Geometry: final body of the model. Coordinates: model frame, mm. Coordinates: 2 decimals unless noted, no trailing zeros. Order: outer loops, then holes, each group sorted by start corner. A loop starts at its lowest first (then second) coordinate and runs counter-clockwise, first axis right, second up. Notation, with made-up numbers: (41, -39.5) -> (50, -39.5) arc R11 cw to (50, -23.5) -> close; hole circle Ø11 at (-22, -8.75). An arc over 180 degrees is marked (long way). Answer in a Markdown table with one row per item. Add a question column.
1) Section query C-C on x = 30. Return the cut outline in (y, z).
2) Section query D-D on y = 174.5. Return the cut outline in (x, z), then the cut area to 3 significant figures.
3) Ray query, line 1 (Y direction, x = 7, z = 4.55); line 2 (X direction, y = 161.5, z = 2.9); line 3 (X direction, y = 85, z = 3.6). Return the intervals inside material, ascending. Write a range as from..to.
4) Section query B-B on x = -4. Return the cut outline in (y, z).
5) Section query A-A on y = 145. Return the cut outline in (x, z).
```python
from build123d import *

# Parameters (mm, degrees)
SKETCH1_W           = 70
SKETCH1_H           = 130
SKETCH1_W_2         = 5
SKETCH1_H_2         = 25
SKETCH1_W_3         = 5.5
SKETCH1_H_3         = 34.894660298
BOSS_EXTRUDE1_DEPTH = 5
CUT_EXTRUDE1_REACH  = 205.568
SKETCH2_W           = 4.8
SKETCH2_H           = 8
SKETCH2_H_2         = 30
SKETCH2_W_2         = 8
SKETCH2_H_3         = 2
SKETCH2_W_3         = 20
SKETCH2_W_4         = 12
SKETCH2_H_4         = 22
CUT_EXTRUDE2_REACH  = 205.568
SKETCH4_R           = 0.4


with BuildPart() as part:
    # Sketch1 → Boss-Extrude1 (new body)
    with BuildSketch(Plane.XY):
        with Locations((0, 135.474649456)):
            Rectangle(SKETCH1_W, SKETCH1_H)
        with Locations((0, 184.474649456)):
            Rectangle(SKETCH1_W_2, SKETCH1_H_2, mode=Mode.SUBTRACT)
        with Locations((0, 117.579989158)):
            Rectangle(SKETCH1_W_2, SKETCH1_H_2, mode=Mode.SUBTRACT)
        with Locations((0, 151.027319307)):
            Rectangle(SKETCH1_W_3, SKETCH1_H_3, mode=Mode.SUBTRACT)
    extrude(amount=BOSS_EXTRUDE1_DEPTH)

    # Sketch2 → Cut-Extrude1 (cut, up to next)
    with BuildSketch(Plane.XY.offset(5), mode=Mode.PRIVATE) as cut_extrude1_sk1:
        with Locations((-31, 189.474649456)):
            Rectangle(SKETCH2_W, SKETCH2_H)
    cut_extrude1_tool1 = extrude(cut_extrude1_sk1.sketch, amount=-CUT_EXTRUDE1_REACH, mode=Mode.PRIVATE) & part.part
    # Sketch2 → Cut-Extrude1 (cut, up to next)
    with BuildSketch(Plane.XY.offset(5), mode=Mode.PRIVATE) as cut_extrude1_sk2:
        with Locations((-31, 150.474649456)):
            Rectangle(SKETCH2_W, SKETCH2_H_2)
    cut_extrude1_tool2 = extrude(cut_extrude1_sk2.sketch, amount=-CUT_EXTRUDE1_REACH, mode=Mode.PRIVATE) & part.part
    # Sketch2 → Cut-Extrude1 (cut, up to next)
    with BuildSketch(Plane.XY.offset(5), mode=Mode.PRIVATE) as cut_extrude1_sk3:
        with Locations((-31, 81.474649456)):
            Rectangle(SKETCH2_W, SKETCH2_H)
    cut_extrude1_tool3 = extrude(cut_extrude1_sk3.sketch, amount=-CUT_EXTRUDE1_REACH, mode=Mode.PRIVATE) & part.part
    # Sketch2 → Cut-Extrude1 (cut, up to next)
    with BuildSketch(Plane.XY.offset(5), mode=Mode.PRIVATE) as cut_extrude1_sk4:
        with Locations((31, 81.474649456)):
            Rectangle(SKETCH2_W, SKETCH2_H)
    cut_extrude1_tool4 = extrude(cut_extrude1_sk4.sketch, amount=-CUT_EXTRUDE1_REACH, mode=Mode.PRIVATE) & part.part
    # Sketch2 → Cut-Extrude1 (cut, up to next)
    with BuildSketch(Plane.XY.offset(5), mode=Mode.PRIVATE) as cut_extrude1_sk5:
        with Locations((31, 150.474649456)):
            Rectangle(SKETCH2_W, SKETCH2_H_2)
    cut_extrude1_tool5 = extrude(cut_extrude1_sk5.sketch, amount=-CUT_EXTRUDE1_REACH, mode=Mode.PRIVATE) & part.part
    # Sketch2 → Cut-Extrude1 (cut, up to next)
    with BuildSketch(Plane.XY.offset(5), mode=Mode.PRIVATE) as cut_extrude1_sk6:
        with Locations((31, 189.474649456)):
            Rectangle(SKETCH2_W, SKETCH2_H)
    cut_extrude1_tool6 = extrude(cut_extrude1_sk6.sketch, amount=-CUT_EXTRUDE1_REACH, mode=Mode.PRIVATE) & part.part
    # Sketch2 → Cut-Extrude1 (cut, up to next)
    with BuildSketch(Plane.XY.offset(5), mode=Mode.PRIVATE) as cut_extrude1_sk7:
        Polygon((10, 196.974649456), (10, 198.974649456), (-10, 198.974649456), (-10, 196.974649456), (-2.5, 196.974649456), (2.5, 196.974649456), align=None)
    cut_extrude1_tool7 = extrude(cut_extrude1_sk7.sketch, amount=-CUT_EXTRUDE1_REACH, mode=Mode.PRIVATE) & part.part
    # Sketch2 → Cut-Extrude1 (cut, up to next)
    with BuildSketch(Plane.XY.offset(5), mode=Mode.PRIVATE) as cut_extrude1_sk8:
        with Locations((29.4, 197.974649456)):
            Rectangle(SKETCH2_W_2, SKETCH2_H_3)
    cut_extrude1_tool8 = extrude(cut_extrude1_sk8.sketch, amount=-CUT_EXTRUDE1_REACH, mode=Mode.PRIVATE) & part.part
    # Sketch2 → Cut-Extrude1 (cut, up to next)
    with BuildSketch(Plane.XY.offset(5), mode=Mode.PRIVATE) as cut_extrude1_sk9:
        with Locations((-29.4, 197.974649456)):
            Rectangle(SKETCH2_W_2, SKETCH2_H_3)
    cut_extrude1_tool9 = extrude(cut_extrude1_sk9.sketch, amount=-CUT_EXTRUDE1_REACH, mode=Mode.PRIVATE) & part.part
    # Sketch2 → Cut-Extrude1 (cut, up to next)
    with BuildSketch(Plane.XY.offset(5), mode=Mode.PRIVATE) as cut_extrude1_sk10:
        with Locations((-29.4, 72.974649456)):
            Rectangle(SKETCH2_W_2, SKETCH2_H_3)
    cut_extrude1_tool10 = extrude(cut_extrude1_sk10.sketch, amount=-CUT_EXTRUDE1_REACH, mode=Mode.PRIVATE) & part.part
    # Sketch2 → Cut-Extrude1 (cut, up to next)
    with BuildSketch(Plane.XY.offset(5), mode=Mode.PRIVATE) as cut_extrude1_sk11:
        with Locations((0, 72.974649456)):
            Rectangle(SKETCH2_W_3, SKETCH2_H_3)
    cut_extrude1_tool11 = extrude(cut_extrude1_sk11.sketch, amount=-CUT_EXTRUDE1_REACH, mode=Mode.PRIVATE) & part.part
    # Sketch2 → Cut-Extrude1 (cut, up to next)
    with BuildSketch(Plane.XY.offset(5), mode=Mode.PRIVATE) as cut_extrude1_sk12:
        with Locations((29.4, 72.974649456)):
            Rectangle(SKETCH2_W_2, SKETCH2_H_3)
    cut_extrude1_tool12 = extrude(cut_extrude1_sk12.sketch, amount=-CUT_EXTRUDE1_REACH, mode=Mode.PRIVATE) & part.part
    # Sketch2 → Cut-Extrude1 (cut, up to next)
    with BuildSketch(Plane.XY.offset(5), mode=Mode.PRIVATE) as cut_extrude1_sk13:
        with Locations((10, 95.474649456)):
            Rectangle(SKETCH2_W_4, SKETCH2_H_4)
    cut_extrude1_tool13 = extrude(cut_extrude1_sk13.sketch, amount=-CUT_EXTRUDE1_REACH, mode=Mode.PRIVATE) & part.part
    add(cut_extrude1_tool1.solids().sort_by_distance((-31, 189.474649, 5))[0], mode=Mode.SUBTRACT)
    add(cut_extrude1_tool2.solids().sort_by_distance((-31, 150.474649, 5))[0], mode=Mode.SUBTRACT)
    add(cut_extrude1_tool3.solids().sort_by_distance((-31, 81.474649, 5))[0], mode=Mode.SUBTRACT)
    add(cut_extrude1_tool4.solids().sort_by_distance((31, 81.474649, 5))[0], mode=Mode.SUBTRACT)
    add(cut_extrude1_tool5.solids().sort_by_distance((31, 150.474649, 5))[0], mode=Mode.SUBTRACT)
    add(cut_extrude1_tool6.solids().sort_by_distance((31, 189.474649, 5))[0], mode=Mode.SUBTRACT)
    add(cut_extrude1_tool7.solids().sort_by_distance((0, 197.974649, 5))[0], mode=Mode.SUBTRACT)
    add(cut_extrude1_tool8.solids().sort_by_distance((29.4, 197.974649, 5))[0], mode=Mode.SUBTRACT)
    add(cut_extrude1_tool9.solids().sort_by_distance((-29.4, 197.974649, 5))[0], mode=Mode.SUBTRACT)
    add(cut_extrude1_tool10.solids().sort_by_distance((-29.4, 72.974649, 5))[0], mode=Mode.SUBTRACT)
    add(cut_extrude1_tool11.solids().sort_by_distance((0, 72.974649, 5))[0], mode=Mode.SUBTRACT)
    add(cut_extrude1_tool12.solids().sort_by_distance((29.4, 72.974649, 5))[0], mode=Mode.SUBTRACT)
    add(cut_extrude1_tool13.solids().sort_by_distance((10, 95.474649, 5))[0], mode=Mode.SUBTRACT)

    # Sketch4 → Cut-Extrude2 (cut, up to next)
    with BuildSketch(Plane.XY.offset(5), mode=Mode.PRIVATE) as cut_extrude2_sk1:
        with Locations((10, 81.974649456)):
            Circle(SKETCH4_R)
    cut_extrude2_tool1 = extrude(cut_extrude2_sk1.sketch, amount=-CUT_EXTRUDE2_REACH, mode=Mode.PRIVATE) & part.part
    # Sketch4 → Cut-Extrude2 (cut, up to next)
    with BuildSketch(Plane.XY.offset(5), mode=Mode.PRIVATE) as cut_extrude2_sk2:
        with Locations((10, 108.974649456)):
            Circle(SKETCH4_R)
    cut_extrude2_tool2 = extrude(cut_extrude2_sk2.sketch, amount=-CUT_EXTRUDE2_REACH, mode=Mode.PRIVATE) & part.part
    add(cut_extrude2_tool1.solids().sort_by_distance((10, 81.974649, 5))[0], mode=Mode.SUBTRACT)
    add(cut_extrude2_tool2.solids().sort_by_distance((10, 108.974649, 5))[0], mode=Mode.SUBTRACT)


solid = part.part
```
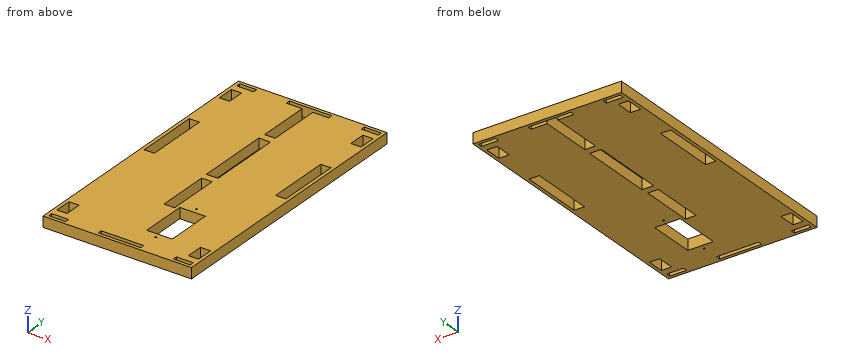
Result:
| question | item | result |
|---|---|---|
| 1 | outline | (70.47, 0) -> (71.97, 0) -> (71.97, 5) -> (70.47, 5) -> close; (73.97, 0) -> (77.47, 0) -> (77.47, 5) -> (73.97, 5) -> close; (85.47, 0) -> (135.47, 0) -> (135.47, 5) -> (85.47, 5) -> close; (165.47, 0) -> (185.47, 0) -> (185.47, 5) -> (165.47, 5) -> close; (193.47, 0) -> (196.97, 0) -> (196.97, 5) -> (193.47, 5) -> close; (198.97, 0) -> (200.47, 0) -> (200.47, 5) -> (198.97, 5) -> close |
| 2 | outline | (-35, 0) -> (-2.5, 0) -> (-2.5, 5) -> (-35, 5) -> close; (2.5, 0) -> (35, 0) -> (35, 5) -> (2.5, 5) -> close |
| 2 | area | 325 mm2 |
| 3 | line 1 | 70.47..71.97, 73.97..84.47, 106.47..196.97, 198.97..200.47 |
| 3 | line 2 | -35..-33.4, -28.6..-2.75, 2.75..28.6, 33.4..35 |
| 3 | line 3 | -35..-33.4, -28.6..4, 16..28.6, 33.4..35 |
| 4 | outline | (70.47, 0) -> (71.97, 0) -> (71.97, 5) -> (70.47, 5) -> close; (73.97, 0) -> (196.97, 0) -> (196.97, 5) -> (73.97, 5) -> close; (198.97, 0) -> (200.47, 0) -> (200.47, 5) -> (198.97, 5) -> close |
| 5 | outline | (-35, 0) -> (-33.4, 0) -> (-33.4, 5) -> (-35, 5) -> close; (-28.6, 0) -> (-2.75, 0) -> (-2.75, 5) -> (-28.6, 5) -> close; (2.75, 0) -> (28.6, 0) -> (28.6, 5) -> (2.75, 5) -> close; (33.4, 0) -> (35, 0) -> (35, 5) -> (33.4, 5) -> close |
